Verification items for the finished model (mm, model axes). Face numbers are marked on the shaded views. Round coordinates to 2 decimals unless told otherwise and drop trailing zeros. Order: outer loops, then holes, each group sorted by start corner. A loop starts at its lowest first (then second) coordinate and runs counter-clockwise, first axis right, second up. Notation, with made-up numbers: M 69.5,52 L 99.5,52 A21 ccw 99.5,69 Z; hole C 24.5,38 d1. An arc over 180 degrees is marked long. Write item = value, one per line. Start each with the question number.
from build123d import *

# Parameters (mm, degrees)
SKETCH1_W           = 76.2
SKETCH1_H           = 25.4
SKETCH1_R           = 2.794
BOSS_EXTRUDE1_DEPTH = 6.35
SKETCH2_W           = 76.2
SKETCH2_H           = 5.08
BOSS_EXTRUDE2_DEPTH = 19.05
SKETCH3_R           = 3.429
CUT_EXTRUDE1_DEPTH  = 5.08


with BuildPart() as part:
    # Sketch1 → Boss-Extrude1 (new body)
    with BuildSketch(Plane(origin=(0, 0, 0), x_dir=(1, 0, 0), z_dir=(0, 1, 0))):
        with Locations((38.1, 12.7)):
            Rectangle(SKETCH1_W, SKETCH1_H)
        with Locations(Location((63.5, 12.7, 0), (0, 0, 270))):
            Circle(SKETCH1_R, mode=Mode.SUBTRACT)
        with Locations(Location((12.7, 12.7, 0), (0, 0, 270))):
            Circle(SKETCH1_R, mode=Mode.SUBTRACT)
    extrude(amount=BOSS_EXTRUDE1_DEPTH)

    # Sketch2 → Boss-Extrude2 (add)
    with BuildSketch(Plane(origin=(0, 6.35, 0), x_dir=(1, 0, 0), z_dir=(0, 1, 0))):
        with Locations((38.1, 2.54)):
            Rectangle(SKETCH2_W, SKETCH2_H)
    extrude(amount=BOSS_EXTRUDE2_DEPTH)

    # Sketch3 → Cut-Extrude1 (cut)
    with BuildSketch(Plane.XY):
        with Locations((38.1, 12.7)):
            Circle(SKETCH3_R)
    extrude(amount=-CUT_EXTRUDE1_DEPTH, mode=Mode.SUBTRACT)


solid = part.part
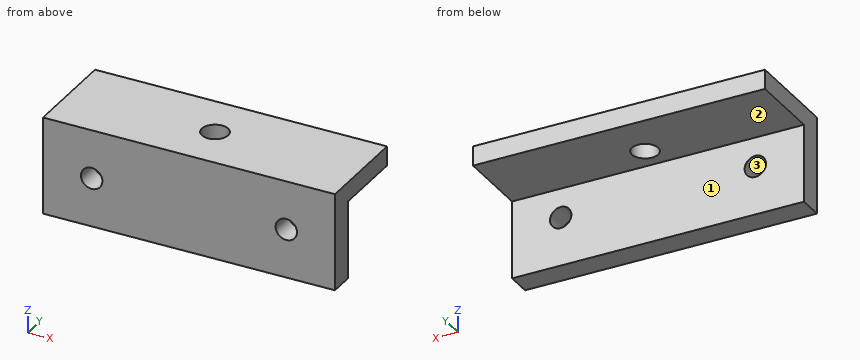
1) Cross-section at C-C, the plane x = 12.7. Enter the section's corners in (y, z).
2) Cross-section at D-D, the plane z = -12.7. Enter the section's corners in (x, y), then the cut area to 3 significant figures.
3) Scan lines: probe 1 along X at (y, z) = (3.25, -12.7); probe 2 along Y at (x, z) = (38.1, -1.7); probe 3 along Y at (x, z) = (47.5, -9.75). Record each from-to range of solid material in increasing order.
4) Gauge pin test, flat ends, axial feed: P1, Ø1, axis at x = 51, y = 16.5, coming from the -Z side; P2, Ø2, axis at x = 61, z = -12.5, coming from the +Y side. Record the tip position at first contact, or that the pin passes through.
5) Release check for a two-part mould opening along Z. For the marked faces 1, 2 and 3 record: pulls with the +Z half, pulls with the -Z half, needs draft (parallel to the pull), parting line crosses it, or undercut.
6) Cross-section at B-B, the plane z = -3.5. Enter the section's corners in (x, y), then the cut area to 3 significant figures.
7) Cross-section at A-A, the plane y = 12.7. Enter the section's corners in (x, z).
Geometry results:
q1.outline = M 0,-25.4 L 6.35,-25.4 L 6.35,-15.49 L 0,-15.49 Z; M 0,-9.91 L 6.35,-9.91 L 6.35,-5.08 L 25.4,-5.08 L 25.4,0 L 0,0 Z
q2.outline = M 0,0 L 9.91,0 L 9.91,6.35 L 0,6.35 Z; M 15.49,0 L 60.71,0 L 60.71,6.35 L 15.49,6.35 Z; M 66.29,0 L 76.2,0 L 76.2,6.35 L 66.29,6.35 Z
q2.area = 413 mm^2
q3.probe_1 = 0 to 9.91, 15.49 to 60.71, 66.29 to 76.2
q3.probe_2 = 0 to 9.27, 16.13 to 25.4
q3.probe_3 = 0 to 6.35
q4.P1 = -5.08
q4.P2 = 6.35
q5.face_1 = needs draft
q5.face_2 = pulls with the -Z half
q5.face_3 = undercut
q6.outline = M 0,0 L 76.2,0 L 76.2,25.4 L 0,25.4 Z; hole C 38.1,12.7 d6.86
q6.area = 1,900 mm^2
q7.outline = M 0,-5.08 L 34.67,-5.08 L 34.67,0 L 0,0 Z; M 41.53,-5.08 L 76.2,-5.08 L 76.2,0 L 41.53,0 Z
